Verification items for this drawing (mm, ordinates from the low corner). A direction names the side the tool comes from. Coordinates: 2 decimals unless noted, no trailing zeros. Write each loop counter-clockwise with the first axis right and the second up, starting at its lowest first coordinate (ties: lowest second). Pieces come first, ordered by that corner, then holes. Notation, with made-up numbers: (70, 2) -> (81, 2) arc R35 ccw to (81, 37) -> close; hole circle Ø7 at (-26, 37). An arc over 180 degrees is marked (long way). One line per question, with ' | ' between items.
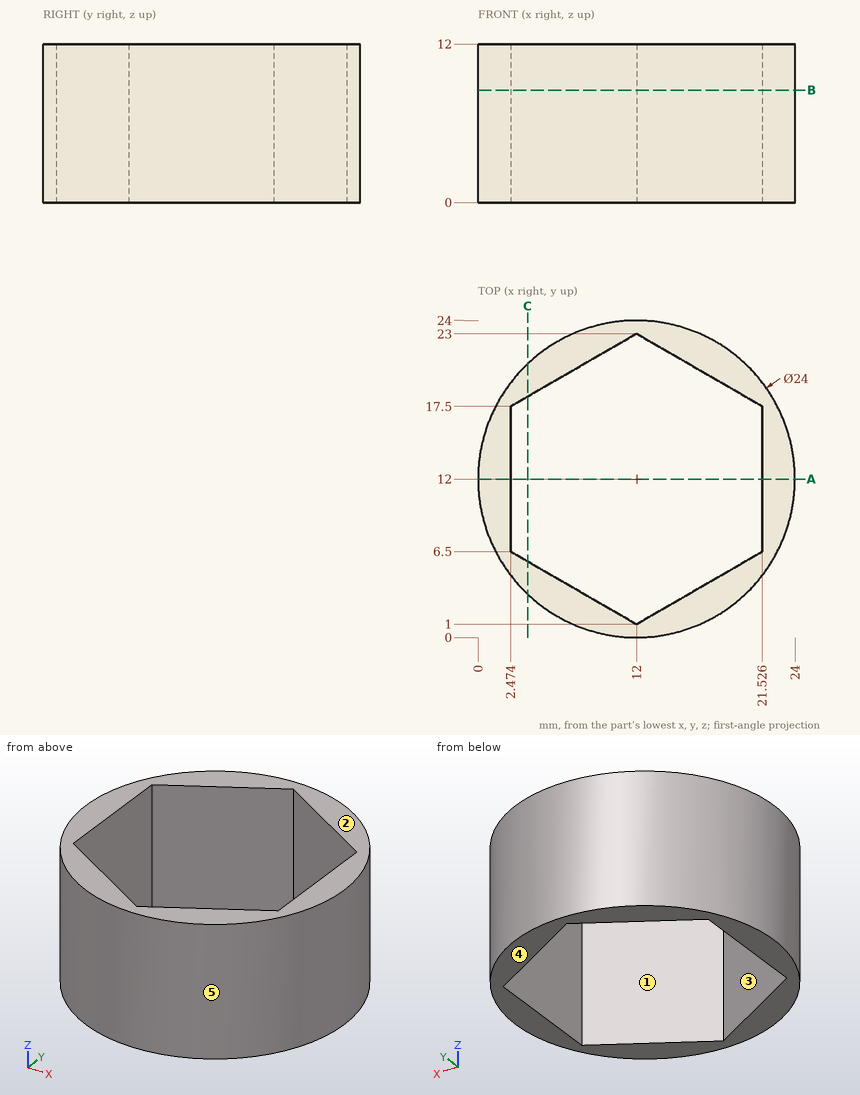
(1) Draft check along X on the marked faces 3, 4 and 5. Enter one of: pulls with the +X half, pulls with the -X half, needs draft (parallel to the pull), parting line crosses it, or undercut.
Answers below:
face 3: undercut | face 4: needs draft | face 5: parting line crosses it
(2) Depth check by flat-ended pin: P1, Ø5, axis at x = 7.5, y = 16, coming from the -Z side (3 decimals); P2, Ø2, axis at y = 4.5, z = 5.5, coming from the +X side; P3, Ø4, axis at y = 6, z = 8.5, coming from the -X side; P4, Ø3, axis at y = 16.5, z = 8, coming from the -X side. Enter the tip coordinate at first touch or a pass-through.
Answers below:
P1: passes through | P2: stops at x = 22.09 | P3: stops at x = 0.69 | P4: stops at x = 0.38
(3) Cross-section at A-A (y = 12). Record the cut outline in (x, z).
Answers below:
outline: (0, 0) -> (2.47, 0) -> (2.47, 12) -> (0, 12) -> close; (21.53, 0) -> (24, 0) -> (24, 12) -> (21.53, 12) -> close
(4) Tool access check on the marked faces 1 and 2. Record the directions out of +Z, -Z, +X, -X, +Y, -Y that give a thin tool (end or side, any length) a straight path to the whole face; none if there is none.
Answers below:
face 1: +Z, -Z | face 2: +Z, +X, -X, +Y, -Y
(5) Cross-section at B-B (z = 8.5). Record the cut outline in (x, y), plus the area to 3 significant figures.
Answers below:
outline: circle Ø24 at (12, 12); hole (2.47, 6.5) -> (12, 1) -> (21.53, 6.5) -> (21.53, 17.5) -> (12, 23) -> (2.47, 17.5) -> close | area: 138 mm²
(6) Cross-section at C-C (x = 3.75). Record the cut outline in (y, z).
Answers below:
outline: (3.29, 0) -> (5.76, 0) -> (5.76, 12) -> (3.29, 12) -> close; (18.24, 0) -> (20.71, 0) -> (20.71, 12) -> (18.24, 12) -> close
(7) Material ranges on line 1 (X direction, y = 21.5, z = 2.5); line 2 (Y direction, x = 15.25, z = 1.75); line 3 (X direction, y = 4, z = 2.25) (1 decimal), recorded low to high.
Answers below:
line 1: x = 4.67 to 9.4, 14.6 to 19.33 | line 2: y = 0.45 to 2.88, 21.12 to 23.55 | line 3: x = 3.1 to 6.8, 17.2 to 20.9
